Autodesk Inventor part; units mm, degrees
ref_plane "YZ Plane" through (0, 0, 0) normal (1, 0, 0) x (0, 1, 0)
ref_plane "XZ Plane" through (0, 0, 0) normal (0, 1, 0) x (-1, 0, 0)
ref_plane "XY Plane" through (0, 0, 0) normal (0, 0, 1) x (1, 0, 0)
sketch "Sketch1" plane through (0, 0, 0) normal (0, 0, 1) x (1, 0, 0)
  line L0 (0, 0) -> (-151, 0)
  line L1 (-151, 0) -> (-151, 112)
  line L2 (-151, 112) -> (0, 112)
  line L3 (0, 112) -> (0, 0)
  line L4 (-151, 0) -> (0, 0)
  line L5 (0, 0) -> (0, -1)
  line L6 (0, -1) -> (-151, -1)
  line L7 (-151, -1) -> (-151, 0)
  dimension "d0" = 151
  dimension "d1" = 112
  dimension "d35" = 1
extrude "Extrusion1" add sketch "Sketch1" along normal blind 3
sketch "Sketch2" plane through (0, 0, 3) normal (0, 0, 1) x (1, 0, 0)
  line L0 (-151, 0) -> (0, 0)
  line L1 (0, 0) -> (-151, 0)
  line L2 (-151, 0) -> (-151, 53)
  line L3 (-151, 53) -> (0, 53)
  line L4 (0, 53) -> (0, 0)
  line L5 (-148, 50) -> (-3, 50)
  line L6 (-3, 50) -> (-3, 3)
  line L7 (-3, 3) -> (-148, 3)
  line L8 (-148, 3) -> (-148, 50)
  line L9 (-151, -1) -> (0, -1)
  line L10 (-151, 112) -> (-151, -1)
  line L11 (0, -1) -> (0, 112)
  line L12 (-148, 3) -> (-3, 3)
  line L13 (-3, 3) -> (-3, 2)
  line L14 (-3, 2) -> (-148, 2)
  line L15 (-148, 2) -> (-148, 3)
  dimension "d4" = 151
  dimension "d5" = 53
  dimension "d6" = 3
  dimension "d7" = 3
  dimension "d8" = 3
  dimension "d9" = 3
  dimension "d36" = 1
extrude "Extrusion2" add sketch "Sketch2" along normal blind 30
sketch "Sketch3" plane through (0, 0, 3) normal (0, 0, 1) x (1, 0, 0)
  line L0 (-148, 109) -> (-103.5, 109)
  line L1 (-103.5, 109) -> (-103.5, 56)
  line L2 (-103.5, 56) -> (-148, 56)
  line L3 (-148, 56) -> (-148, 109)
  line L4 (-47.5, 109) -> (-3, 109)
  line L5 (-3, 109) -> (-3, 56)
  line L6 (-3, 56) -> (-47.5, 56)
  line L7 (-47.5, 56) -> (-47.5, 109)
  line L8 (0, 112) -> (-151, 112)
  line L9 (-151, 112) -> (-151, 53)
  line L10 (0, 53) -> (0, 112)
  line L11 (-85.5, 100) -> (-65.5, 100)
  line L12 (-65.5, 100) -> (-65.5, 65)
  line L13 (-65.5, 65) -> (-85.5, 65)
  line L14 (-85.5, 65) -> (-85.5, 100)
  line L15 (-62.5, 103) -> (-88.5, 103)
  line L16 (-88.5, 103) -> (-88.5, 62)
  line L17 (-88.5, 62) -> (-62.5, 62)
  line L18 (-62.5, 62) -> (-62.5, 103)
  line L19 (-100.5, 112) -> (-151, 112)
  line L20 (-151, 112) -> (-151, 53)
  line L21 (-151, 53) -> (-100.5, 53)
  line L22 (-100.5, 53) -> (-100.5, 112)
  line L23 (0, 112) -> (-50.5, 112)
  line L24 (-50.5, 112) -> (-50.5, 53)
  line L25 (-50.5, 53) -> (0, 53)
  line L26 (0, 53) -> (0, 112)
  point P0 (0, 0)
  dimension "d12" = 44.5
  dimension "d13" = 53
  dimension "d14" = 44.5
  dimension "d15" = 53
  dimension "d16" = 3
  dimension "d17" = 3
  dimension "d18" = 3
  dimension "d19" = 20
  dimension "d20" = 35
  dimension "d21" = 12
  dimension "d22" = 18
  dimension "d23" = 3
  dimension "d24" = 3
  dimension "d25" = 3
extrude "Extrusion3" add sketch "Sketch3" along normal blind 8
fillet "Fillet1" radius 4 6 edges at (-100.5, 82.5, 3) (-62.5, 82.5, 3) (-50.5, 82.5, 3) (-75.5, 103, 3) (-88.5, 82.5, 3) (-75.5, 62, 3)
sketch "Sketch6" plane through (-151, -1, 0) normal (0, -1, 0) x (1, 0, 0)
  line L0 (65.5, 21) -> (85.5, 21)
  line L1 (85.5, 21) -> (85.5, 18)
  line L2 (85.5, 18) -> (65.5, 18)
  line L3 (65.5, 18) -> (65.5, 21)
  line L4 (0, 0) -> (0, 33)
  line L5 (0, 33) -> (151, 33)
  point P0 (151, 0)
  dimension "d37" = 20
  dimension "d38" = 3
  dimension "d39" = 65.5
  dimension "d40" = 12
extrude "Extrusion5" cut sketch "Sketch6" against normal up to surface (54 mm away)
sketch "Sketch7" plane through (0, 0, 11) normal (0, 0, 1) x (1, 0, 0)
  line L0 (0, 112) -> (-151, 112)
  line L1 (0, 112) -> (-151, 112)
  line L2 (-151, 112) -> (-151, 53)
  line L3 (-151, 53) -> (0, 53)
  line L4 (0, 53) -> (0, 112)
  point P0 (0, 0)
extrude "Extrusion6" cut sketch "Sketch7" against normal up to surface (11 mm away)
sketch "Sketch8" plane through (-151, -1, 0) normal (-1, 0, 0) x (0, 0, 1)
  arc A0 (38.3305, 78.7131) -> (30.8341, -23.2131) centre (44.5445, 27.0173) ccw
  line L0 (10, 65.9756) -> (10, -11.9409)
  line L1 (10, 65.9756) -> (87.9165, 65.9756) construction
  line L2 (0, 54) -> (33, 54)
  line L3 (0, 0) -> (33, 0)
  point P0 (0, 1)
  point P1 (0.0136, 54)
  point P2 (10, 54)
  point P3 (10, 0)
  point P4 (0.0346, 0)
  dimension "d45" = 90
extrude "Extrusion7" add sketch "Sketch8" against normal up to surface (151 mm away) contours L0 L2 A0 | L3 L0 A0
properties part number "bateria_mocowanie_ramie_robota"
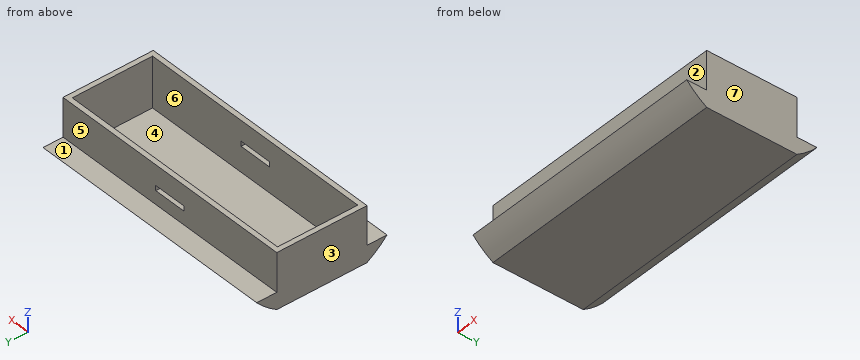
Could you check a few things on this model? Use its own coordinates, in mm. Face numbers are marked on the shaded views. A direction names the side the tool comes from. Coordinates: 2 decimals unless noted, no trailing zeros. Order: outer loops, then holes, each group sorted by start corner. A loop starts at its lowest first (then second) coordinate and runs counter-clockwise, first axis right, second up.
Q1. Will these pins go through, and if not, where does the flat tip stop? pin 1 (10 mm diameter, centred on x = -119.5, z = 25.5, fed in from -Y); pin 2 (1.5 mm diameter, centred on x = -127.5, y = 16, fed in from +Z); pin 3 (18.5 mm diameter, centred on x = -66, z = 20, fed in from +Y).
Q2. Suppose I cut it at A-A on z = 13. Please give me the cut outline in (x, y), and give its area (3 significant figures).
Q3. Suppose I cut it at B-B on y = 25.5. Please give me the cut outline in (x, z).
Q4. Thinking about a two-plate mould opening in X: for the marked faces 5, 6 and 7, which applies, released by +X, released by -X, zero draft, split by the parting line, or undercut?
Q5. Please list where these lines run through material, in increasing order: L1, parallel to Y at x = -95, z = 25.5; L2, parallel to X at y = 17, z = 29.5; L3, parallel to Z at x = -23.5, y = 33.
Q6. Which directions (+Z, -Z, +X, -X, +Y, -Y) give clear straight access to the entire face, cutting with the end or side of a thin tool? Please do the marked faces 1, 2, 3 and 4.
Q7. Suppose I cut it at C-C on x = -77.5. Give the number of separate pieces and of enclosed holes in the cut face, and give its area (3 significant figures).
Answer:
1. pin 1: stops at y = -1
1. pin 2: stops at z = 3
1. pin 3: stops at y = 53
2. outline: (-151, -1) - (0, -1) - (0, 53) - (-151, 53) - close; hole (-148, 2) - (-3, 2) - (-3, 50) - (-148, 50) - close
2. area: 1,190 mm2
3. outline: (-151, 0) - (0, 0) - (0, 33) - (-3, 33) - (-3, 3) - (-148, 3) - (-148, 33) - (-151, 33) - close
4. face 5: zero draft
4. face 6: undercut
4. face 7: released by +X
5. L1: y = -1 to 2, 50 to 53
5. L2: x = -151 to -148, -3 to 0
5. L3: z = 0 to 3
6. face 1: +Z, +X, -X, +Y
6. face 2: +Z, +X, -X, -Y
6. face 3: +Z, -Z, -X, +Y, -Y
6. face 4: +Z
7. separate pieces: 3
7. enclosed holes: 0
7. area: 455 mm2
